Build history of the part. All positions in model axes, mm. A direction names the side the tool comes from. Coordinates: 2 decimals unless noted, no trailing zeros. Loops run counter-clockwise (first coordinate to the right, second up) from the corner with the lowest first, then second, coordinate; pieces in that order, holes last.
(1) Two-plate mould, pull along X, no slides. Class faces 6 (the face through (-44, 14, 3.2)), 7 (the face through (-28.37, 5.4, 5.27)), 8 (the face through (-33, 0, 7.4)), 9 (the face through (-58.622, 20, 2)): pulls with the +X half, pulls with the -X half, needs draft (parallel to the pull), parting line crosses it, or undercut.
(2) Slice it at C-C (z = 6). Give the cut face in (x, y), and give its area (3 significant figures).
(3) Slice it at B-B (x = -41). Give the cut face in (y, z).
(4) Slice it at D-D (z = 2). Give the cut face in (x, y).
(5) Slice it at A-A (y = -16). Give the cut face in (x, z).
(6) Flat gauge pins, fed straight in: P1, Ø10.5, axis at x = -29, y = -28, coming from the -Z side; P2, Ø1.3, axis at x = -37.5, z = 6, coming from the -Y side; P3, Ø1.9, axis at x = -43, y = 4, coming from the +Z side. Where does each tip first touch, or does it go through?
(7) Wall check: L1, parallel to Z at x = -23, y = -26; L2, parallel to X at y = -37, z = 4; L3, parallel to Y at x = -33, z = 2.25. Give the ranges that are in metal, low to high.
(8) Tool access for faces 1 (the face through (-42.09, -35, 5)), 2 (the face through (-44, 0, 2)), 3 (the face through (-37, -39.753, 5)), 4 (the face through (-43, 2, 3.2)), 5 (the face through (-52.4, -21.9, 5.3)): list every direction of +Z, -Z, +X, -X, +Y, -Y with a clear straight run to the whole face (end or side of a thin tool).
from build123d import *

# Parameters (mm, degrees)
F0_W     = 30
F0_H     = 40
F1_DEPTH = 3.2
F2_R     = 5.11227941
F3_DEPTH = 25
F5_DEPTH = 4.2


with BuildPart() as f1:
    # F0 (on Top) → F1 (new body)
    with BuildSketch(Plane.XY):
        with Locations((-43.6224012077, 20)):
            Rectangle(F0_W, F0_H)
    extrude(amount=F1_DEPTH)

    # F2 (on face) → F3 (cut)
    with BuildSketch(Plane.XY.offset(3.2)):
        with Locations((-43.6224012077, 13.6897208655)):
            Circle(F2_R)
    extrude(amount=-F3_DEPTH, mode=Mode.SUBTRACT)

    # F4 (on face) → F5 (join)
    with BuildSketch(Plane.XY.offset(3.2)):
        Polygon((-60.0767214389, -13.6426556282), (-67.4975478184, -5.6577981007), (-72.8724002838, -12.7526037395), (-65.8724009991, -20.2526040375), align=None)
        Polygon((-50.7815668435, 16.4072979817), (-67.4975478184, -5.6577981007), (-60.0767214389, -13.6426556282), (-42.700756127, 6.1745604691), align=None)
        Polygon((-52.4952933192, 18.5773912817), (-50.7815668435, 16.4072979817), (-47.8724017739, 20.2473960817), (-35.6223993003, 14.2473969609), (-42.700756127, 6.1745604691), (-23.0845756663, -18.6654256037), (-15.3557008339, -12.9879858125), (-15.0352679193, -12.7526037395), (-42.0897305012, 24.077475071), align=None)
        Polygon((-47.8724017739, 20.2473960817), (-50.7815668435, 16.4072979817), (-42.700756127, 6.1745604691), (-35.6223993003, 14.2473969609), align=None)
        Polygon((-44.8723994195, -30.00260517), (-60.0767214389, -13.6426556282), (-65.8724009991, -20.2526040375), (-50.1223988831, -39.7526025772), (-44.8723994195, -40.2526035905), align=None)
        Polygon((-15.3557008339, -12.9879858125), (-23.0845756663, -18.6654256037), (-42.0897305012, -30.00260517), (-42.0897305012, -39.7526025772), (-31.8723991513, -39.7526025772), (-7.6223979704, -20.2526040375), align=None)
    extrude(amount=F5_DEPTH)


solid = f1.part
Response values:
1. face 6: undercut
1. face 7: pulls with the +X half
1. face 8: needs draft
1. face 9: pulls with the -X half
2. outline: (-72.87, -12.75) - (-65.87, -20.25) - (-50.12, -39.75) - (-44.87, -40.25) - (-44.87, -30) - (-60.08, -13.64) - (-42.7, 6.17) - (-23.08, -18.67) - (-42.09, -30) - (-42.09, -39.75) - (-31.87, -39.75) - (-7.62, -20.25) - (-15.36, -12.99) - (-15.04, -12.75) - (-42.09, 24.08) - (-52.5, 18.58) - (-50.78, 16.41) - close
2. area: 1,590 mm2
3. outline: (-39.75, 3.2) - (-29.35, 3.2) - (-29.35, 7.4) - (-39.75, 7.4) - close; (0, 0) - (9.3, 0) - (9.3, 3.2) - (18.08, 3.2) - (18.08, 0) - (40, 0) - (40, 3.2) - (22.59, 3.2) - (22.59, 7.4) - (4.02, 7.4) - (4.02, 3.2) - (0, 3.2) - close
4. outline: (-58.62, 0) - (-28.62, 0) - (-28.62, 40) - (-58.62, 40) - close; hole circle Ø10.22 at (-43.62, 13.69)
5. outline: (-69.84, 3.2) - (-57.89, 3.2) - (-57.89, 7.4) - (-69.84, 7.4) - close; (-25.19, 3.2) - (-12.15, 3.2) - (-12.15, 7.4) - (-25.19, 7.4) - close
6. P1: stops at z = 3.2
6. P2: stops at y = -39.75
6. P3: stops at z = 3.2
7. L1: z = 3.2 to 7.4
7. L2: x = -52.35 to -44.87, -42.09 to -28.45
7. L3: y = 0 to 40
8. face 1: +Z, -Z, -Y
8. face 2: -Z, +X, -X, -Y
8. face 3: +Z, -Z, +X, -Y
8. face 4: +Z
8. face 5: +Z, -Z
